Geometry check sheet. Reference: the model listing, model coordinates, mm. Face numbers are marked on the shaded views. A direction names the side the tool comes from. Give positions to 0.01 mm unless a question says otherwise; leave off trailing zeros. Loops run counter-clockwise (first coordinate to the right, second up) from the corner with the lowest first, then second, coordinate; pieces in that order, holes last. Notation, with made-up numbers: (-40, 18.25) - (6, 18.25) arc R26 ccw to (6, 54.25) - close; hole circle Ø6 at (57, 35). An arc over 180 degrees is marked (long way). Write item = value, one per line. Start each with the question number.
from build123d import *

# Parameters (mm, degrees)
IZIM3_W                     = 15.52
IZIM3_H                     = 8.1
Y_KSEKLIK_EKSTR_ZYON1_DEPTH = 2.13
Y_KSEKLIK_EKSTR_ZYON2_DEPTH = 4.55
KES_EKSTR_ZYON2_DEPTH       = 12.275
KES_EKSTR_ZYON3_DEPTH       = 12.275
KES_EKSTR_ZYON4_DEPTH       = 16.52
IZIM10_R                    = 3.505
IZIM10_R_2                  = 1.155
Y_KSEKLIK_EKSTR_ZYON4_DEPTH = 0.775
IZIM11_R                    = 1.155
Y_KSEKLIK_EKSTR_ZYON5_DEPTH = 4.215


with BuildPart() as part:
    # Çizim3 → Yükseklik-Ekstrüzyon1 (new body)
    with BuildSketch(Plane(origin=(0, 0, 0), x_dir=(1, 0, 0), z_dir=(0, 1, 0))):
        with Locations((-7.76, -4.05)):
            Rectangle(IZIM3_W, IZIM3_H)
    extrude(amount=-Y_KSEKLIK_EKSTR_ZYON1_DEPTH)

    # Çizim4 → Yükseklik-Ekstrüzyon2 (add)
    with BuildSketch(Plane(origin=(0, 0, 0), x_dir=(1, 0, 0), z_dir=(0, 1, 0))):
        with BuildLine():
            Line((-13.045, -1.61), (-10.265, -1.61))
            ThreePointArc((-10.265, -1.61), (-10.017011641, -2.32335475), (-9.38, -2.729050937))
            Line((-9.38, -2.729050937), (-9.38, -5.370949063))
            ThreePointArc((-9.38, -5.370949063), (-10.017011641, -5.77664525), (-10.265, -6.49))
            Line((-10.265, -6.49), (-13.045, -6.49))
            ThreePointArc((-13.045, -6.49), (-13.292988359, -5.77664525), (-13.93, -5.370949063))
            Line((-13.93, -5.370949063), (-13.93, -2.729050937))
            ThreePointArc((-13.93, -2.729050937), (-13.292988359, -2.32335475), (-13.045, -1.61))
        make_face()
        with BuildLine():
            Line((-6.14, -2.729050937), (-6.14, -5.370949063))
            ThreePointArc((-6.14, -5.370949063), (-5.502988359, -5.77664525), (-5.255, -6.49))
            Line((-5.255, -6.49), (-2.475, -6.49))
            ThreePointArc((-2.475, -6.49), (-2.227011641, -5.77664525), (-1.59, -5.370949063))
            Line((-1.59, -5.370949063), (-1.59, -2.729050937))
            ThreePointArc((-1.59, -2.729050937), (-2.227011641, -2.32335475), (-2.475, -1.61))
            Line((-2.475, -1.61), (-5.255, -1.61))
            ThreePointArc((-5.255, -1.61), (-5.502988359, -2.32335475), (-6.14, -2.729050937))
        make_face()
    extrude(amount=Y_KSEKLIK_EKSTR_ZYON2_DEPTH)

    # Çizim6 → Kes-Ekstrüzyon2 (cut, symmetric)
    with BuildSketch(Plane.XY.offset(5.370949063)):
        Polygon((-1.59, 1.68), (-1.59, 4.55), (-2.148911229, 4.55), align=None)
    extrude(amount=KES_EKSTR_ZYON2_DEPTH, both=True, mode=Mode.SUBTRACT)

    # Çizim7 → Kes-Ekstrüzyon3 (cut, symmetric)
    with BuildSketch(Plane.XY.offset(5.370949063)):
        Polygon((-13.93, 4.55), (-13.371088771, 4.55), (-13.93, 1.68), align=None)
    extrude(amount=KES_EKSTR_ZYON3_DEPTH, both=True, mode=Mode.SUBTRACT)

    # Çizim8 → Kes-Ekstrüzyon4 (cut, through all)
    with BuildSketch(Plane(origin=(0, 0, 0), x_dir=(0, 0, -1), z_dir=(1, 0, 0))):
        with BuildLine():
            ThreePointArc((-6.78, -2.13), (-4.05, -1.267106893), (-1.32, -2.13))
            Line((-1.32, -2.13), (-6.78, -2.13))
        make_face()
    extrude(amount=-KES_EKSTR_ZYON4_DEPTH, mode=Mode.SUBTRACT)

    # Çizim10 → Yükseklik-Ekstrüzyon4 (add, symmetric)
    with BuildSketch(Plane(origin=(-7.76, 0, 0), x_dir=(0, 0, -1), z_dir=(1, 0, 0))):
        with BuildLine():
            Line((-6.78, -2.13), (-6.78, -2.661790501))
            ThreePointArc((-6.78, -2.661790501), (-4.05, -1.355), (-1.32, -2.661790501))
            Line((-1.32, -2.661790501), (-1.32, -2.13))
            ThreePointArc((-1.32, -2.13), (-4.05, -1.267106893), (-6.78, -2.13))
        make_face()
        with Locations((-4.05, -4.86)):
            Circle(IZIM10_R)
        with Locations((-4.05, -4.86)):
            Circle(IZIM10_R_2, mode=Mode.SUBTRACT)
    extrude(amount=Y_KSEKLIK_EKSTR_ZYON4_DEPTH, both=True)

    # Çizim11 → Yükseklik-Ekstrüzyon5 (add, symmetric)
    with BuildSketch(Plane(origin=(-7.76, 0, 0), x_dir=(0, 0, -1), z_dir=(1, 0, 0))):
        with Locations((-4.05, -4.86)):
            Circle(IZIM11_R)
    extrude(amount=Y_KSEKLIK_EKSTR_ZYON5_DEPTH, both=True)


solid = part.part
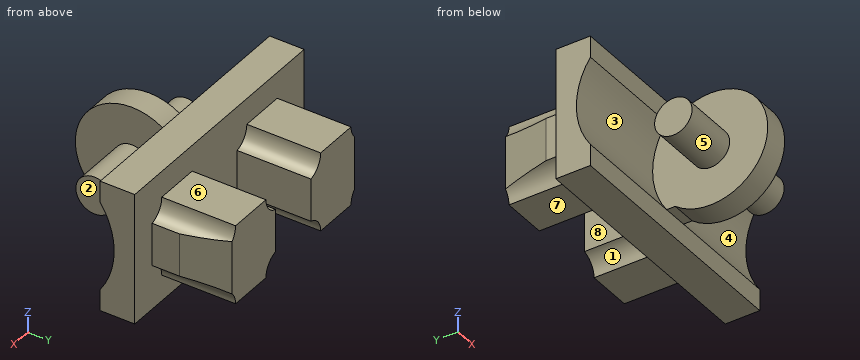
1) Material ranges on line 1 along X through (y, z) = (1.5, 4.5); line 2 along X through (y, z) = (-3.5, 2) (3 decimals); line 3 along Y through (x, z) = (-10.25, 4.75), recorded low to high.
2) Cross-section at B-B on y = 3.5. Enter the section's corners in (x, z) (3 decimals).
3) Tool access check on the marked faces 4, 5, 6, 7 and 8. Record the directions out of +Z, -Z, +X, -X, +Y, -Y that give a thin tool (end or side, any length) a straight path to the whole face; none if there is none.
4) Cross-section at D-D on x = -8.25. Enter the section's corners in (y, z) (3 decimals), and give its area (3 significant figures).
5) Gauge pin test, flat ends, axial feed: P1, Ø3, axis at x = -3.5, y = 2.5, coming from the +Z side; P2, Ø0.5, axis at y = 0.5, z = 4, coming from the +X side; P3, Ø1, axis at x = -5.5, y = 3, coming from the -Z side; P4, Ø6, axis at x = -11.5, y = -3, coming from the +Z side. Record the tip position at first contact, or that the pin passes through.
6) Cross-section at A-A on x = -11.75. Enter the section's corners in (y, z) (3 decimals), and give its area (3 significant figures).
7) Release check for a two-part mould opening along Z. For the marked faces 1, 2 and 3 record: pulls with the +Z half, pulls with the -Z half, needs draft (parallel to the pull), parting line crosses it, or undercut.
8) Cross-section at C-C on z = 4.05. Enter the section's corners in (x, y) (3 decimals).
Checked values:
q1.line_1 = -13.93 to -9.38, -6.14 to -1.59
q1.line_2 = -8.535 to -6.985
q1.line_3 = -5.78 to -3.94, -1.32 to 4.55
q2.outline = (-13.576, 2.579) arc R1.15 cw to (-13.045, 1.61) - (-10.265, 1.61) arc R1.15 cw to (-9.38, 2.729) - (-9.38, 5.371) arc R1.15 cw to (-10.265, 6.49) - (-13.045, 6.49) arc R1.15 cw to (-13.576, 5.521) - close; (-6.14, 2.729) arc R1.15 cw to (-5.255, 1.61) - (-2.475, 1.61) arc R1.15 cw to (-1.944, 2.579) - (-1.944, 5.521) arc R1.15 cw to (-2.475, 6.49) - (-5.255, 6.49) arc R1.15 cw to (-6.14, 5.371) - close
q3.face_4 = +X
q3.face_5 = -X
q3.face_6 = +Z, +X, -X, +Y
q3.face_7 = -Z, +X, -X, +Y
q3.face_8 = +Z, -Z, +Y
q4.outline = (-2.662, 1.32) - (-2.13, 1.32) - (-2.13, 0) - (0, 0) - (0, 8.1) - (-2.13, 8.1) - (-2.13, 6.78) - (-2.662, 6.78) arc R3.505 ccw (long way) to start
q4.area = 53.8 mm²
q5.P1 = 6.49
q5.P2 = -1.59
q5.P3 = 1.61
q5.P4 = 8.1
q6.outline = circle Ø2.31 at (-4.86, 4.05); (-2.13, 0) - (0, 0) - (0, 1.61) - (4.55, 1.61) - (4.55, 6.49) - (0, 6.49) - (0, 8.1) - (-2.13, 8.1) - (-2.13, 6.78) arc R4.75 cw to (-2.13, 1.32) - close
q6.area = 40.4 mm²
q7.face_1 = pulls with the -Z half
q7.face_2 = needs draft
q7.face_3 = undercut
q8.outline = (-15.52, -1.267) - (-8.535, -1.267) - (-8.535, -3.705) - (-11.975, -3.705) - (-11.975, -6.015) - (-8.535, -6.015) - (-8.535, -8.365) - (-6.985, -8.365) - (-6.985, -6.015) - (-3.545, -6.015) - (-3.545, -3.705) - (-6.985, -3.705) - (-6.985, -1.267) - (0, -1.267) - (0, 0) - (-1.59, 0) - (-1.59, 1.68) - (-2.149, 4.55) - (-6.14, 4.55) - (-6.14, 0) - (-9.38, 0) - (-9.38, 4.55) - (-13.371, 4.55) - (-13.93, 1.68) - (-13.93, 0) - (-15.52, 0) - close
